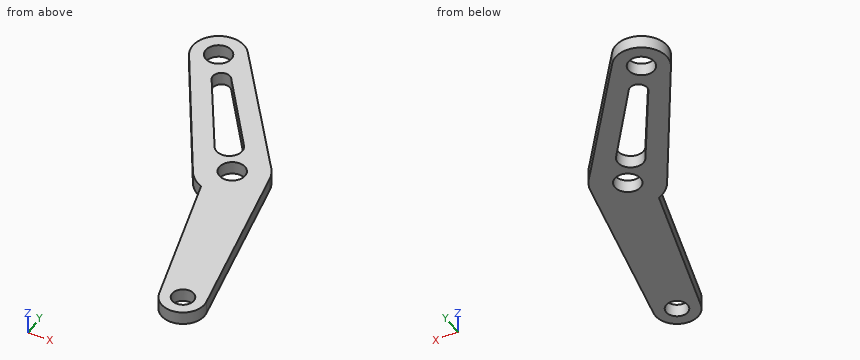
```python
from build123d import *

# Parameters (mm, degrees)
SKETCH_2_R      = 2.5
SKETCH_2_R_2    = 3
EXTRUDE_1_DEPTH = 3


with BuildPart() as part:
    # 草图2 → 凸台-拉伸1 (new body)
    with BuildSketch(Plane.XY):
        with BuildLine():
            Line((-37.947439952, 28.393304212), (-18.983503384, -4.475664586))
            ThreePointArc((-18.983503384, -4.475664586), (-17.391534203, -6.436907823), (-15.267421048, -7.804015799))
            Line((-15.267421048, -7.804015799), (-6.013345572, -42.340695651))
            ThreePointArc((-6.013345572, -42.340695651), (-0.063044856, -45.919391741), (3.726011827, -40.100784195))
            Line((3.726011827, -40.100784195), (-4.198551107, 1.035590248))
            ThreePointArc((-4.198551107, 1.035590248), (-4.715435995, 2.707212985), (-5.583372683, 4.226482041))
            Line((-5.583372683, 4.226482041), (-27.897341927, 34.919914183))
            ThreePointArc((-27.897341927, 34.919914183), (-36.018233875, 36.423789268), (-37.947439952, 28.393304212))
        make_face()
        with Locations((-1.18371644, -41.046600426)):
            Circle(SKETCH_2_R, mode=Mode.SUBTRACT)
        with Locations((-12.054116335, -0.477715722)):
            Circle(SKETCH_2_R_2, mode=Mode.SUBTRACT)
        with Locations((-32.750399665, 31.39176586)):
            Circle(SKETCH_2_R_2, mode=Mode.SUBTRACT)
        with BuildLine():
            Line((-30.118407474, 23.670491895), (-18.998908748, 4.713784689))
            ThreePointArc((-18.998908748, 4.713784689), (-14.77731151, 3.715637118), (-13.9720864, 7.978241292))
            Line((-13.9720864, 7.978241292), (-26.767192575, 25.846796296))
            ThreePointArc((-26.767192575, 25.846796296), (-29.482565455, 26.359742452), (-30.118407474, 23.670491895))
        make_face(mode=Mode.SUBTRACT)
    extrude(amount=EXTRUDE_1_DEPTH)


solid = part.part
```
Build history of the part. All positions in model axes, mm. Round coordinates to 2 decimals unless told otherwise and drop trailing zeros. Write each loop counter-clockwise with the first axis right and the second up, starting at its lowest first coordinate (ties: lowest second). Pieces come first, ordered by that corner, then holes. Notation, with made-up numbers: (63, 56.25) - (77, 56.25) arc R18 cw to (77, 76.25) - close; hole circle Ø4 at (16, -2.5). An arc over 180 degrees is marked (long way). Write each question's results on one line, items separated by ' | '. Start each with the question number.
Item 1: Saw through at D-D (y = -18). Write the cut outline in (x, z), and give its area (3 significant figures).
Item 2: Saw through at A-A (x = 0). Write the cut outline in (y, z), and give its area (3 significant figures).
Item 3: Saw through at B-B (y = 29.5). Write the cut outline in (x, z).
Item 4: Drop flat-ended pins along their axis: P1, Ø8, axis at x = -32.75, y = 31.39, coming from the -Z side; P2, Ø1, axis at x = -28, z = 0.5, coming from the -Y side. Give the stop position or say it passes through.
Item 5: Wall check: L1, parallel to X at y = -42, z = 0.9; L2, parallel to X at y = 12.5, z = 0.9; L3, parallel to Y at x = -24.5, z = 2.75. Give the ranges that are in metal, low to high. Write a range as [from, to].
Item 6: Saw through at C-C (z = 1.25). Write the cut outline in (x, y), and give its area (3 significant figures).
Results are:
1) outline: (-12.54, 0) - (-0.53, 0) - (-0.53, 3) - (-12.54, 3) - close | area: 36.0 mm²
2) outline: (-45.9, 0) - (-43.25, 0) - (-43.25, 3) - (-45.9, 3) - close; (-38.84, 0) - (-20.76, 0) - (-20.76, 3) - (-38.84, 3) - close | area: 62.2 mm²
3) outline: (-38.44, 0) - (-35.08, 0) - (-35.08, 3) - (-38.44, 3) - close; (-30.42, 0) - (-23.96, 0) - (-23.96, 3) - (-30.42, 3) - close
4) P1: stops at z = 0 | P2: stops at y = 10.29
5) L1: x = [-6.1, -3.49], [1.13, 3.72] | L2: x = [-28.78, -23.57], [-17.21, -11.6] | L3: y = [5.09, 14.09], [22.68, 30.25]
6) outline: (-37.95, 28.39) - (-18.98, -4.48) arc R8 ccw to (-15.27, -7.8) - (-6.01, -42.34) arc R5 ccw to (3.73, -40.1) - (-4.2, 1.04) arc R8 ccw to (-5.58, 4.23) - (-27.9, 34.92) arc R6 ccw to start; hole circle Ø6 at (-32.75, 31.39); hole (-30.12, 23.67) - (-19, 4.71) arc R3 ccw (long way) to (-13.97, 7.98) - (-26.77, 25.85) arc R2 ccw to start; hole circle Ø6 at (-12.05, -0.48); hole circle Ø5 at (-1.18, -41.05) | area: 919 mm²
